Answer from the drawing. Dimensions are ordinates in mm from the lowest x, y and z of the part. Coordinates: 2 decimals unless noted, no trailing zeros. Write each loop counter-clockwise with the first axis right and the second up, starting at its lowest first coordinate (ties: lowest second). Pieces come first, ordered by that corner, then holes. Notation, with made-up numbers: (39.25, 65.25) - (59.25, 65.25) arc R12 cw to (59.25, 74.25) - close; hole circle Ø4 at (47.5, -16.5). An arc over 180 degrees is marked (long way). Return JSON: item names as keys, results as strings.
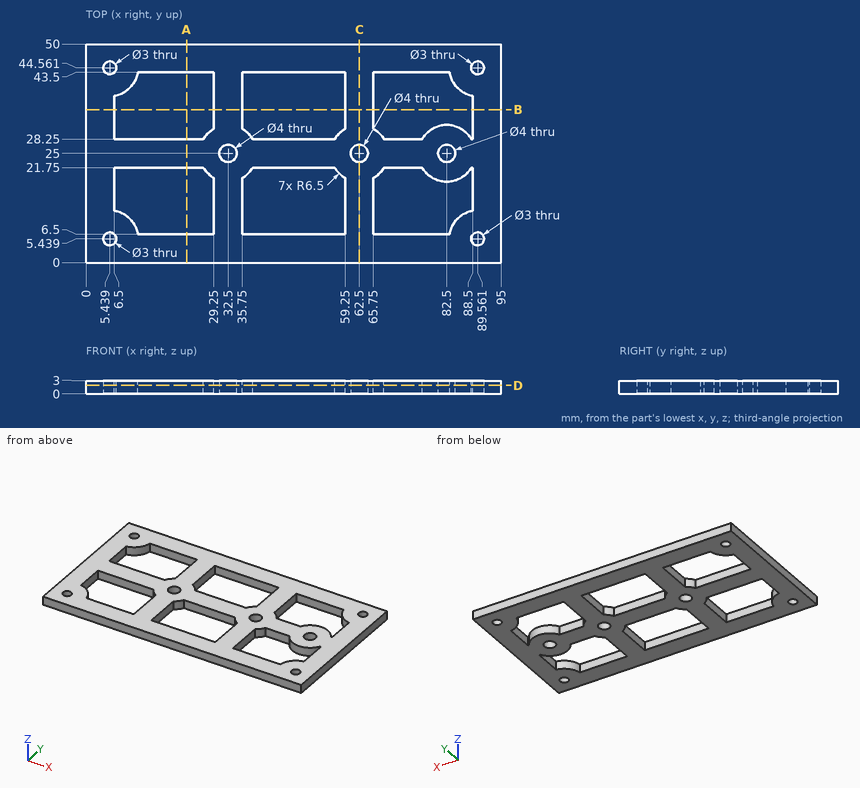
(1) A cutting plane is placed at D-D (z = 1.9). State how many separate pieces and enclosed holes the cut face has, and give its area (3 significant figures).
Answer:
{"separate pieces": "1", "enclosed holes": "13", "area": "2,740 mm²"}
(2) A cutting plane is placed at A-A (x = 23). Determine the outline of the cut face in (y, z).
Answer:
{"outline": "(0, 0) - (6.5, 0) - (6.5, 3) - (0, 3) - close; (21.75, 0) - (28.25, 0) - (28.25, 3) - (21.75, 3) - close; (43.5, 0) - (50, 0) - (50, 3) - (43.5, 3) - close"}
(3) Straight lines are drawn through the part: line 1 (X direction, y = 12.5, z = 1.55); line 2 (Y direction, x = 13, z = 0.6); line 3 (X direction, y = 25, z = 1.8). For each, find the intervals that lie inside material, in ascending order. Write a range as from..to.
Answer:
{"line 1": "0..6.5, 29.25..35.75, 59.25..65.75, 88.5..95", "line 2": "0..6.5, 21.75..28.25, 43.5..50", "line 3": "0..30.5, 34.5..60.5, 64.5..80.5, 84.5..95"}
(4) A cutting plane is placed at C-C (x = 62.5). Determine the outline of the cut face in (y, z), and give its area (3 significant figures).
Answer:
{"outline": "(0, 0) - (23, 0) - (23, 3) - (0, 3) - close; (27, 0) - (50, 0) - (50, 3) - (27, 3) - close", "area": "138 mm²"}
(5) A cutting plane is placed at B-B (y = 35). Determine the outline of the cut face in (x, z).
Answer:
{"outline": "(0, 0) - (6.5, 0) - (6.5, 3) - (0, 3) - close; (29.25, 0) - (35.75, 0) - (35.75, 3) - (29.25, 3) - close; (59.25, 0) - (65.75, 0) - (65.75, 3) - (59.25, 3) - close; (88.5, 0) - (95, 0) - (95, 3) - (88.5, 3) - close"}
